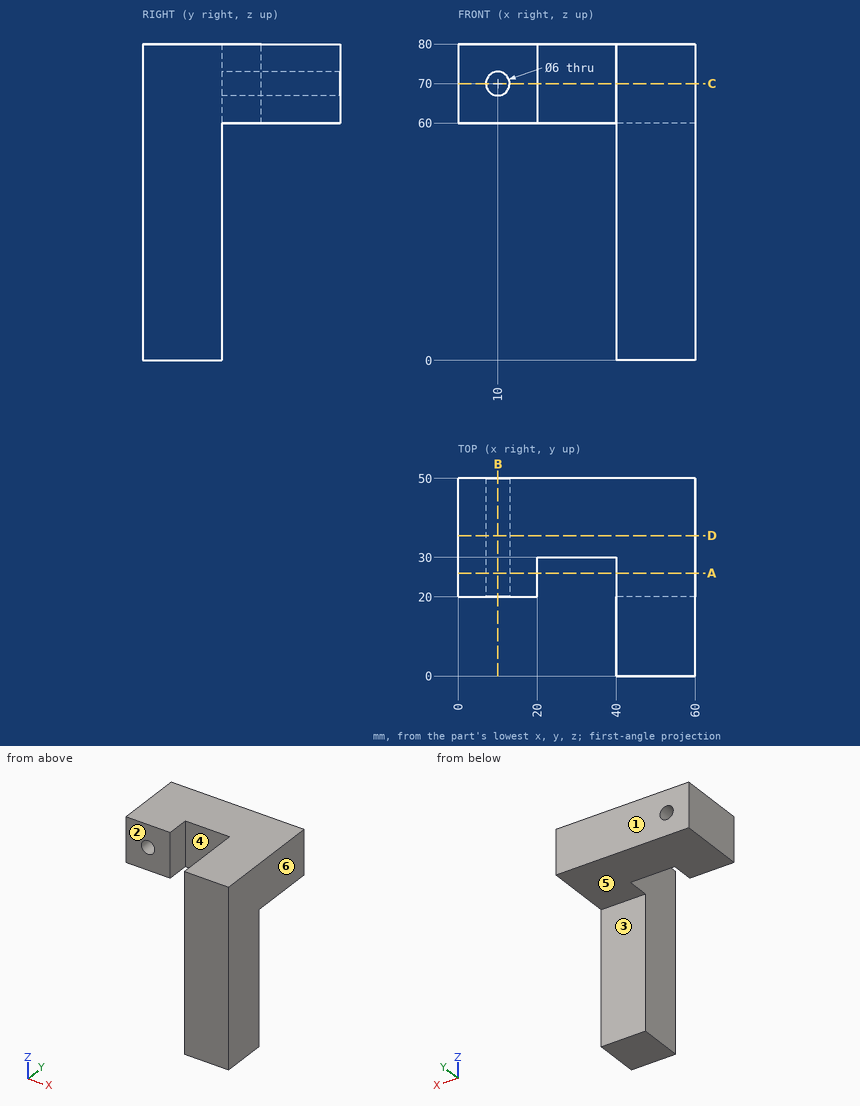
Job drawing, mm, ordinate dimensions from the low corner. One solid piece. A direction names the side the tool comes from. Round coordinates to 2 decimals unless told otherwise and drop trailing zeros. Loops run counter-clockwise (first coordinate to the right, second up) from the corner with the lowest first, then second, coordinate; pieces in that order, holes last. Notation, with made-up numbers: M 16.5,8.5 L 68.5,8.5 A12 ccw 68.5,25.5 Z; hole C 55,9.25 d1. An arc over 180 degrees is marked long. One line per question, with ' | ' between items. Start each with the question number.
Item 1: Pin check, flat tips, straight feed: pin 1 Ø15 at (y, z) = (22, 27) entering from -X; pin 2 Ø15 at (x, y) = (32.5, 39.5) entering from -Z; pin 3 Ø6 at (x, z) = (47, 31) entering from +Y. Stop position of each tip, or through.
Item 2: Cut at D-D, the plane y = 35.5. Write the cut outline in (x, z).
Item 3: Two-plate mould, pull along X, no slides. Class the marked faces 4, 5 and 6: pulls with the +X half, pulls with the -X half, needs draft (parallel to the pull), parting line crosses it, or undercut.
Item 4: Cut at A-A, the plane y = 26. Write the cut outline in (x, z), plus the area to 3 significant figures.
Item 5: Which spindle directions (+Z, -Z, +X, -X, +Y, -Y) get a long thin tool onto all of the face, cutting with end or side? Do the marked faces 1, 2 and 3. Say none if no direction does.
Item 6: Wall check: line 1 (X direction, y = 29, z = 70); line 2 (X direction, y = 34, z = 70); line 3 (Y direction, x = 42, z = 21). Give the ranges that are in metal, low to high.
Item 7: Cut at B-B, the plane x = 10. Write the cut outline in (y, z), plus the area to 3 significant figures.
Item 8: Cut at C-C, the plane z = 70. Write the cut outline in (x, y), plus the area to 3 significant figures.
Responses:
1) pin 1: stops at x = 40 | pin 2: stops at z = 60 | pin 3: stops at y = 20
2) outline: M 0,60 L 60,60 L 60,80 L 0,80 Z; hole C 10,70 d6
3) face 4: undercut | face 5: needs draft | face 6: pulls with the +X half
4) outline: M 0,60 L 20,60 L 20,80 L 0,80 Z; M 40,60 L 60,60 L 60,80 L 40,80 Z; hole C 10,70 d6 | area: 772 mm²
5) face 1: +Z, -Z, +X, -X, +Y | face 2: +Z, -Z, -X, -Y | face 3: -Z, +X, -X, +Y
6) line 1: x = 0 to 7, 13 to 20, 40 to 60 | line 2: x = 0 to 7, 13 to 60 | line 3: y = 0 to 20
7) outline: M 20,60 L 50,60 L 50,67 L 20,67 Z; M 20,73 L 50,73 L 50,80 L 20,80 Z | area: 420 mm²
8) outline: M 0,20 L 7,20 L 7,50 L 0,50 Z; M 13,20 L 20,20 L 20,30 L 40,30 L 40,0 L 60,0 L 60,50 L 13,50 Z | area: 1,820 mm²
